from build123d import *

# Parameters (mm, degrees)
SKETCH1_W           = 190
SKETCH1_H           = 220
BOSS_EXTRUDE1_DEPTH = 120
CHAMFER1_SIZE       = 40
CHAMFER2_SIZE       = 15
SHELL1_T            = -3


with BuildPart() as part:
    # Sketch1 → Boss-Extrude1 (new body)
    with BuildSketch(Plane(origin=(0, 0, 0), x_dir=(1, 0, 0), z_dir=(0, 1, 0))):
        Rectangle(SKETCH1_W, SKETCH1_H)
    extrude(amount=BOSS_EXTRUDE1_DEPTH)

    # Chamfer1
    chamfer1_edges = [part.edges().sort_by_distance(p)[0] for p in [
        (-95, 120, 0),
        (0, 120, 110),
        (95, 120, 0),
        (0, 120, -110),
    ]]
    chamfer(chamfer1_edges, length=CHAMFER1_SIZE)

    # Chamfer2
    chamfer2_edges = [part.edges().sort_by_distance(p)[0] for p in [
        (95, 40, 110),
        (-95, 40, 110),
        (-95, 40, -110),
        (95, 40, -110),
    ]]
    chamfer(chamfer2_edges, length=CHAMFER2_SIZE)

    # Shell1
    shell1_openings = [part.faces().sort_by_distance(p)[0] for p in [
        (0, 0, 0),
    ]]
    offset(amount=SHELL1_T, openings=shell1_openings, kind=Kind.INTERSECTION)


solid = part.part
Source: CAD feature listing. Evaluate the final solid. Frame: model axes, mm. A direction names the side the tool comes from. Coordinates: 2 decimals unless noted, no trailing zeros. Write each loop counter-clockwise with the first axis right and the second up, starting at its lowest first coordinate (ties: lowest second). Pieces come first, ordered by that corner, then holes. Notation, with made-up numbers: M -1,3 L 34,3 A22 ccw 34,38 Z; hole C 82.5,3 d3. An arc over 180 degrees is marked long. Use a Markdown table: item, result.
1) Ray query, L1, parallel to X at y = 24, z = -42.5; L2, parallel to Z at x = -49, y = 70.5; L3, parallel to Y at x = 20, z = -67.5. Return the intervals inside material, ascending.
Conclusion:
| item | result |
|---|---|
| L1 | x = -95 to -92, 92 to 95 |
| L2 | z = -110 to -107, 107 to 110 |
| L3 | y = 117 to 120 |
2) Section C-C, the plane x = 32.5. Output: boundary loops of the cut face in (y, z), then the cut area to 3 significant figures.
Conclusion:
| item | result |
|---|---|
| outline | M 0,-110 L 80,-110 L 120,-70 L 120,70 L 80,110 L 0,110 L 0,107 L 78.76,107 L 117,68.76 L 117,-68.76 L 78.76,-107 L 0,-107 Z |
| area | 1,220 mm^2 |
3) Section D-D, the plane y = 107. Output: boundary loops of the cut face in (x, z).
Conclusion:
| item | result |
|---|---|
| outline | M -68,-83 L 68,-83 L 68,83 L -68,83 Z; hole M -63.76,-78.76 L 63.76,-78.76 L 63.76,78.76 L -63.76,78.76 Z |
4) Section B-B, the plane z = 65.5. Output: boundary loops of the cut face in (x, y).
Conclusion:
| item | result |
|---|---|
| outline | M -95,0 L -92,0 L -92,78.76 L -53.76,117 L 53.76,117 L 92,78.76 L 92,0 L 95,0 L 95,80 L 55,120 L -55,120 L -95,80 Z |
5) Reachability of faces 1 (the flat face through (92, 39, 1)), 2 (the flat face through (88, 43, -102)) from +Z, -Z, +X, -X, +Y, -Y: full face, straight path, thin tool, end or side. Return the list, or none.
Conclusion:
| item | result |
|---|---|
| face 1 | -Y |
| face 2 | -Z, +X, +Y, -Y |
6) Section A-A, the plane y = 64.5. Output: boundary loops of the cut face in (x, z).
Conclusion:
| item | result |
|---|---|
| outline | M -95,-95 L -80,-110 L 80,-110 L 95,-95 L 95,95 L 80,110 L -80,110 L -95,95 Z; hole M -92,-93.76 L -78.76,-107 L 78.76,-107 L 92,-93.76 L 92,93.76 L 78.76,107 L -78.76,107 L -92,93.76 Z |
7) First-contact query: pin 1 Ø6 at (x, z) = (-71.5, 3.5) entering from -Y; pin 2 Ø10 at (x, z) = (-72, 67) entering from -Y; pin 3 Ø1.5 at (x, y) = (42.5, 81.5) entering from -Z. Flat tips, straight axial feed; report the tip coordinate or a pass-through.
Conclusion:
| item | result |
|---|---|
| pin 1 | stops at y = 96.26 |
| pin 2 | stops at y = 93.76 |
| pin 3 | stops at z = -109.25 |
8) Mould query, pull axis Z, two halves, no side actions, for faces 3 (the flat face through (88, 43, 102)), 4 (the flat face through (-1, 120, -1)), 5 (the flat face through (-1.2, 98.15, -87.61)). Classes: pulls with the +Z half, pulls with the -Z half, needs draft (parallel to the pull), parting line crosses it, or undercut.
Conclusion:
| item | result |
|---|---|
| face 3 | pulls with the +Z half |
| face 4 | needs draft |
| face 5 | undercut |
